CAD build for the part. Positions are in the model's coordinates, mm. Face numbers are marked on the shaded views. A direction names the side the tool comes from. Coordinates: 2 decimals unless noted, no trailing zeros. Order: outer loops, then holes, each group sorted by start corner. A loop starts at its lowest first (then second) coordinate and runs counter-clockwise, first axis right, second up. Notation, with made-up numbers: M 37.25,6 L 78.25,6 A37 ccw 78.25,42 Z; hole C 73.25,0.5 d6. An arc over 180 degrees is marked long. One line per item, written item: value.
from build123d import *

# Parameters (mm, degrees)
SKETCH1_W           = 40
SKETCH1_H           = 20
BOSS_EXTRUDE2_DEPTH = 37.5
SKETCH2_W           = 2
SKETCH2_H           = 20
BOSS_EXTRUDE3_DEPTH = 7.25
SKETCH3_R           = 1.995473195
CUT_EXTRUDE1_DEPTH  = 2
FILLET3_R           = 4
SKETCH4_W           = 2
SKETCH4_H           = 20
BOSS_EXTRUDE4_DEPTH = 7.25
SKETCH5_R           = 2
CUT_EXTRUDE2_DEPTH  = 2
FILLET4_R           = 4
SKETCH6_R           = 4.001263217
BOSS_EXTRUDE5_DEPTH = 1
SKETCH7_R           = 2.001461963
BOSS_EXTRUDE7_DEPTH = 4


with BuildPart() as part:
    # Sketch1 → Boss-Extrude2 (new body)
    with BuildSketch(Plane.XY):
        Rectangle(SKETCH1_W, SKETCH1_H)
    extrude(amount=BOSS_EXTRUDE2_DEPTH)

    # Sketch2 → Boss-Extrude3 (add)
    with BuildSketch(Plane(origin=(20, 0, 0), x_dir=(0, 0, -1), z_dir=(1, 0, 0))):
        with Locations((-31, 0)):
            Rectangle(SKETCH2_W, SKETCH2_H)
    extrude(amount=BOSS_EXTRUDE3_DEPTH)

    # Sketch3 → Cut-Extrude1 (cut)
    with BuildSketch(Plane.XY.offset(32)):
        with Locations((24.75, -4.99913934)):
            Circle(SKETCH3_R)
        with Locations((24.75, 4.999429987)):
            Circle(SKETCH3_R)
    extrude(amount=-CUT_EXTRUDE1_DEPTH, mode=Mode.SUBTRACT)

    # Fillet3
    fillet3_edges = [part.edges().sort_by_distance(p)[0] for p in [
        (27.25, -10, 31),
        (27.25, 10, 31),
    ]]
    fillet(fillet3_edges, radius=FILLET3_R)

    # Sketch4 → Boss-Extrude4 (add)
    with BuildSketch(Plane.ZY.offset(20)):
        with Locations((31, 0)):
            Rectangle(SKETCH4_W, SKETCH4_H)
    extrude(amount=BOSS_EXTRUDE4_DEPTH)

    # Sketch5 → Cut-Extrude2 (cut)
    with BuildSketch(Plane.XY.offset(32)):
        with Locations((-24.75, 5)):
            Circle(SKETCH5_R)
        with Locations((-24.75, -5)):
            Circle(SKETCH5_R)
    extrude(amount=-CUT_EXTRUDE2_DEPTH, mode=Mode.SUBTRACT)

    # Fillet4
    fillet4_edges = [part.edges().sort_by_distance(p)[0] for p in [
        (-27.25, -10, 31),
        (-27.25, 10, 31),
    ]]
    fillet(fillet4_edges, radius=FILLET4_R)

    # Sketch6 → Boss-Extrude5 (add)
    with BuildSketch(Plane.XY.offset(37.5)):
        with Locations((-10, 0)):
            Circle(SKETCH6_R)
    extrude(amount=BOSS_EXTRUDE5_DEPTH)

    # Sketch7 → Boss-Extrude7 (add)
    with BuildSketch(Plane.XY.offset(38.5)):
        with Locations((-10, 0)):
            Circle(SKETCH7_R)
    extrude(amount=BOSS_EXTRUDE7_DEPTH)


solid = part.part
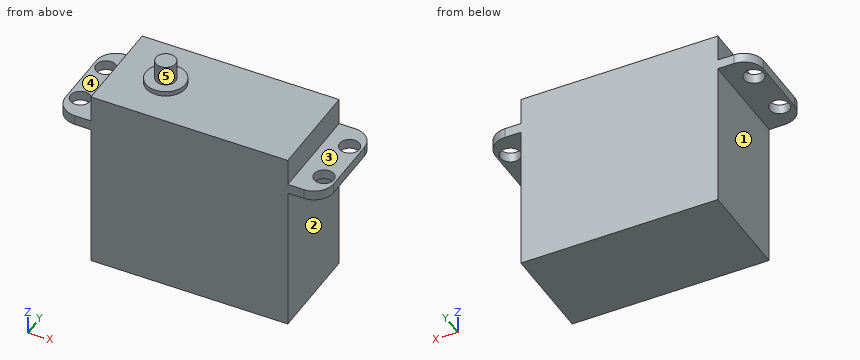
Q1. Pin check, flat tips, straight feed: pin 1 Ø3 at (x, y) = (12.5, 1) entering from -Z; pin 2 Ø2 at (y, z) = (-4, 8.5) entering from -X; pin 3 Ø8 at (x, y) = (-22.5, 1) entering from +Z; pin 4 Ø4.5 at (x, y) = (-24.75, -5) entering from -Z. Stop position of each tip, or through.
Recorded:
pin 1: stops at z = 0
pin 2: stops at x = -20
pin 3: stops at z = 37.5
pin 4: stops at z = 30
Q2. Slice it at C-C (z = 31). List the corners of the cut face in (x, y), plus the area to 3 significant figures.
Recorded:
outline: M -27.25,-6 A4 ccw -23.25,-10 L 23.25,-10 A4 ccw 27.25,-6 L 27.25,6 A4 ccw 23.25,10 L -23.25,10 A4 ccw -27.25,6 Z; hole C -24.75,-5 d4; hole C -24.75,5 d4; hole C 24.75,-5 d3.99; hole C 24.75,5 d3.99
area: 1,030 mm^2
Q3. Slice it at A-A (x = -10). List the corners of the cut face in (y, z).
Recorded:
outline: M -10,0 L 10,0 L 10,37.5 L 4,37.5 L 4,38.5 L 2,38.5 L 2,42.5 L -2,42.5 L -2,38.5 L -4,38.5 L -4,37.5 L -10,37.5 Z
Q4. Drill centre lines: line 1 along Y through (x, z) = (-24.75, 31.3); line 2 along X through (y, z) = (0.5, 17); line 3 along Z through (x, y) = (-9.5, -7.75). Where is each one in solid material? Low to high.
Recorded:
line 1: y = -9.71 to -7, -3 to 3, 7 to 9.71
line 2: x = -20 to 20
line 3: z = 0 to 37.5
Q5. Slice it at B-B (y = 0). List the corners of the cut face in (x, z).
Recorded:
outline: M -27.25,30 L -20,30 L -20,0 L 20,0 L 20,30 L 27.25,30 L 27.25,32 L 20,32 L 20,37.5 L -6,37.5 L -6,38.5 L -8,38.5 L -8,42.5 L -12,42.5 L -12,38.5 L -14,38.5 L -14,37.5 L -20,37.5 L -20,32 L -27.25,32 Z
Q6. Which spindle directions (+Z, -Z, +X, -X, +Y, -Y) get a long thin tool onto all of the face, cutting with end or side? Do the marked faces 1, 2, 3, 4 and 5. Say none if no direction does.
Recorded:
face 1: -Z, -X, +Y, -Y
face 2: -Z, +X, +Y, -Y
face 3: +Z, +X, +Y, -Y
face 4: +Z, -X, +Y, -Y
face 5: +Z
Q7. Slice it at D-D (x = -24.75). List the corners of the cut face in (y, z).
Recorded:
outline: M -9.71,30 L -7,30 L -7,32 L -9.71,32 Z; M -3,30 L 3,30 L 3,32 L -3,32 Z; M 7,30 L 9.71,30 L 9.71,32 L 7,32 Z
